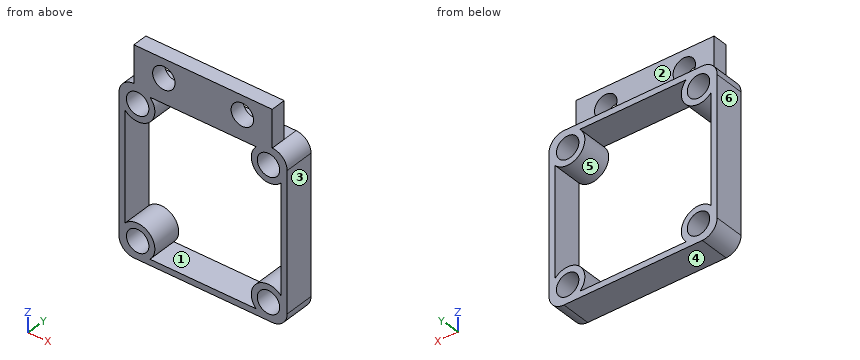
from build123d import *

# Parameters (mm, degrees)
SKETCH1_R           = 1.5
BOSS_EXTRUDE1_DEPTH = 4
SKETCH2_W           = 18.5
SKETCH2_H           = 2
BOSS_EXTRUDE2_DEPTH = 5
SKETCH3_R           = 1.5
CUT_EXTRUDE1_DEPTH  = 5


with BuildPart() as part:
    # Sketch1 → Boss-Extrude1 (new body)
    with BuildSketch(Plane(origin=(0, 0, 0), x_dir=(1, 0, 0), z_dir=(0, 1, 0))):
        with BuildLine():
            Line((-9.25, 11.25), (9.25, 11.25))
            ThreePointArc((9.25, 11.25), (10.664213562, 10.664213562), (11.25, 9.25))
            Line((11.25, 9.25), (11.25, -9.25))
            ThreePointArc((11.25, -9.25), (10.664213562, -10.664213562), (9.25, -11.25))
            Line((9.25, -11.25), (-9.25, -11.25))
            ThreePointArc((-9.25, -11.25), (-10.664213562, -10.664213562), (-11.25, -9.25))
            Line((-11.25, -9.25), (-11.25, 9.25))
            ThreePointArc((-11.25, 9.25), (-10.664213562, 10.664213562), (-9.25, 11.25))
        make_face()
        with Locations(Location((8.75, 8.85, 0), (0, 0, 270))):
            Circle(SKETCH1_R, mode=Mode.SUBTRACT)
        with Locations(Location((8.75, -8.85, 0), (0, 0, 90))):
            Circle(SKETCH1_R, mode=Mode.SUBTRACT)
        with Locations(Location((-8.75, 8.85, 0), (0, 0, 90))):
            Circle(SKETCH1_R, mode=Mode.SUBTRACT)
        with Locations(Location((-8.75, -8.85, 0), (0, 0, 270))):
            Circle(SKETCH1_R, mode=Mode.SUBTRACT)
        with BuildLine():
            Line((-7.097728836, 10.45), (7.097728836, 10.45))
            ThreePointArc((7.097728836, 10.45), (7.175222498, 7.173671924), (10.45, 7.300806662))
            Line((10.45, 7.300806662), (10.45, -7.300806662))
            ThreePointArc((10.45, -7.300806662), (7.175222498, -7.173671924), (7.097728836, -10.45))
            Line((7.097728836, -10.45), (-7.097728836, -10.45))
            ThreePointArc((-7.097728836, -10.45), (-7.175222498, -7.173671924), (-10.45, -7.300806662))
            Line((-10.45, -7.300806662), (-10.45, 7.300806662))
            ThreePointArc((-10.45, 7.300806662), (-7.175222498, 7.173671924), (-7.097728836, 10.45))
        make_face(mode=Mode.SUBTRACT)
    extrude(amount=BOSS_EXTRUDE1_DEPTH)

    # Sketch2 → Boss-Extrude2 (add)
    with BuildSketch(Plane.XY.offset(11.25)):
        with Locations((0, 1)):
            Rectangle(SKETCH2_W, SKETCH2_H)
    extrude(amount=BOSS_EXTRUDE2_DEPTH)

    # Sketch3 → Cut-Extrude1 (cut)
    with BuildSketch(Plane(origin=(0, 2, 0), x_dir=(1, 0, 0), z_dir=(0, 1, 0))):
        with Locations(Location((5.25, -13.75, 0), (0, 0, 270))):
            Circle(SKETCH3_R)
        with Locations(Location((-5.25, -13.75, 0), (0, 0, 90))):
            Circle(SKETCH3_R)
    extrude(amount=-CUT_EXTRUDE1_DEPTH, mode=Mode.SUBTRACT)


solid = part.part
The listing builds one solid part. Answer for the finished solid, in the listing's coordinates (mm). Face numbers are marked on the shaded views. A direction names the side the tool comes from. Round coordinates to 2 decimals unless told otherwise and drop trailing zeros. Write each loop counter-clockwise with the first axis right and the second up, starting at its lowest first coordinate (ties: lowest second). Pieces come first, ordered by that corner, then holes. Notation, with made-up numbers: (67.25, -34.75) - (79.25, -34.75) arc R8 cw to (79.25, -19.75) - close; hole circle Ø11 at (6.5, -28). An arc over 180 degrees is marked (long way). Use a Markdown table: item, result. Add a question column.
1. For a pull along X with two mould halves and no side action, classify the marked faces 4, 5 and 6 as +X half, -X half, draft (parallel to the pull), parting line (faces both ways), or undercut.
2. The part is cut by section B-B (z = 8.85). Write down the section's boundary in (x, y), and give its area (3 significant figures).
3. The part is cut by section C-C (z = -0.5). Write down the section's boundary in (x, y), and give its area (3 significant figures).
4. Flat-ended cylindrical pins translate along their axes: P1, Ø1.6, axis at y = 1.5, z = 12.5, coming from the +X side; P2, Ø1, axis at x = 4, y = 3, coming from the +Z side; P3, Ø1.5, axis at x = 1.5, z = 14.5, coming from the +Y side. Find the tip coordinate at first contact, or state that the pin passes through.
5. A tool of negligible diameter and unlimited length cuts with its end or side. For the marked faces 1, 2 and 3, from which of +Z, -Z, +X, -X, +Y, -Y can it reach the whole face along a straight path? Write none if from no direction.
6. The part is cut by section A-A (x = -3). Write down the section's boundary in (y, z).
7. Consider line 1 (Z direction, x = -5.25, y = 1.35); line 2 (X direction, y = 1.7, z = -8.85); line 3 (X direction, y = 1.6, z = 13.75). Determine where each line is inside the solid, lowest interval first.
8. The part is cut by section D-D (x = 5.25). Write down the section's boundary in (y, z).
Reported:
| question | item | result |
|---|---|---|
| 1 | face 4 | draft |
| 1 | face 5 | undercut |
| 1 | face 6 | -X half |
| 2 | outline | (-11.25, 0) - (-10.25, 0) - (-10.25, 4) - (-11.25, 4) - close; (-7.25, 0) - (-6.45, 0) - (-6.45, 4) - (-7.25, 4) - close; (6.45, 0) - (7.25, 0) - (7.25, 4) - (6.45, 4) - close; (10.25, 0) - (11.25, 0) - (11.25, 4) - (10.25, 4) - close |
| 2 | area | 14.4 mm^2 |
| 3 | outline | (-11.25, 0) - (-10.45, 0) - (-10.45, 4) - (-11.25, 4) - close; (10.45, 0) - (11.25, 0) - (11.25, 4) - (10.45, 4) - close |
| 3 | area | 6.40 mm^2 |
| 4 | P1 | x = 9.25 |
| 4 | P2 | z = 11.25 |
| 4 | P3 | y = 2 |
| 5 | face 1 | +Y, -Y |
| 5 | face 2 | +Z, +X, -X, +Y |
| 5 | face 3 | +Z, -Z, +X, +Y, -Y |
| 6 | outline | (0, -11.25) - (4, -11.25) - (4, -10.45) - (0, -10.45) - close; (0, 10.45) - (4, 10.45) - (4, 11.25) - (2, 11.25) - (2, 16.25) - (0, 16.25) - close |
| 7 | line 1 | -11.25 to -10.45, 10.45 to 12.25, 15.25 to 16.25 |
| 7 | line 2 | -11.25 to -10.25, -7.25 to -6.45, 6.45 to 7.25, 10.25 to 11.25 |
| 7 | line 3 | -9.25 to -6.75, -3.75 to 3.75, 6.75 to 9.25 |
| 8 | outline | (0, -11.25) - (4, -11.25) - (4, -10.45) - (0, -10.45) - close; (0, 10.45) - (4, 10.45) - (4, 11.25) - (2, 11.25) - (2, 12.25) - (0, 12.25) - close; (0, 15.25) - (2, 15.25) - (2, 16.25) - (0, 16.25) - close |
